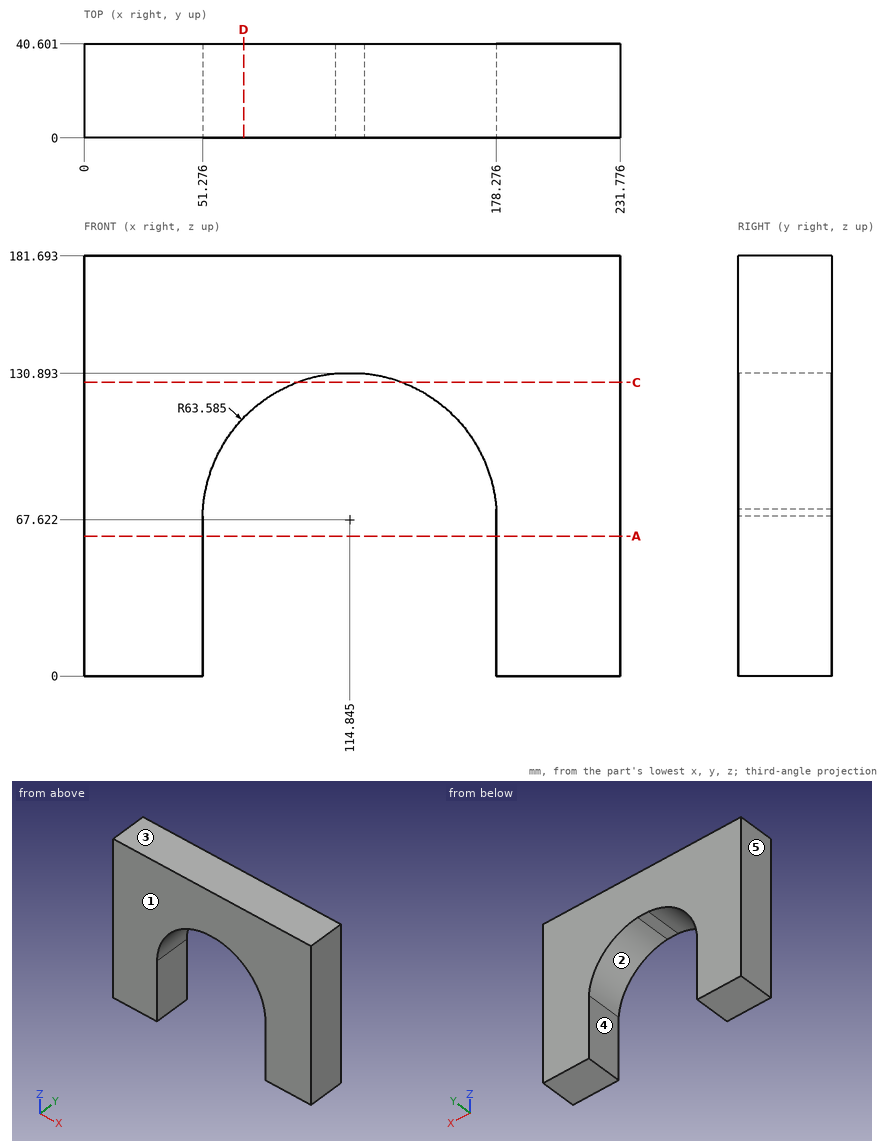
Drawing for the job (mm, zero at the part's lowest x, y, z). A direction names the side the tool comes from. Round coordinates to 2 decimals unless told otherwise and drop trailing zeros. Loops run counter-clockwise (first coordinate to the right, second up) from the corner with the lowest first, then second, coordinate; pieces in that order, holes last.
1. Mould opens along X. For the marked faces 3, 4 and 5 say: +X half, -X half, draft (parallel to the pull), parting line (faces both ways), or undercut.
Check values:
face 3: draft
face 4: undercut
face 5: -X half
2. Drop flat-ended pins along their axis: P1, Ø4, axis at x = 113.5, y = 15, coming from the -Z side; P2, Ø6, axis at x = 66, y = 30, coming from the -Z side (1 decimal). Give the stop position or say it passes through.
Check values:
P1: stops at z = 130.89
P2: stops at z = 104.4
3. Wall check: probe 1 along X at (y, z) = (13.5, 38); probe 2 along X at (y, z) = (19, 113) (1 decimal); probe 3 along Z at (x, y) = (66, 35) (1 decimal). Give the ranges that are in metal, low to high.
Check values:
probe 1: x = 0 to 51.28, 178.28 to 231.78
probe 2: x = 0 to 70.3, 159.4 to 231.8
probe 3: z = 108.3 to 181.7
4. Band-saw the part on C-C, the plane z = 127. List the corners of the cut face in (x, y), and give its area (3 significant figures).
Check values:
outline: (0, 0) - (92.1, 0) - (92.1, 40.6) - (0, 40.6) - close; (137.59, 0) - (231.78, 0) - (231.78, 40.6) - (137.59, 40.6) - close
area: 7,560 mm2
5. Tool access for the marked faces 1 and 2: list every direction of +Z, -Z, +X, -X, +Y, -Y with a clear straight run to the whole face (end or side of a thin tool).
Check values:
face 1: +Z, -Z, +X, -X, -Y
face 2: -Z, +Y, -Y
6. Band-saw the part on A-A, the plane z = 60.5. List the corners of the cut face in (x, y).
Check values:
outline: (0, 0) - (51.28, 0) - (51.28, 40.6) - (0, 40.6) - close; (178.28, 0) - (231.78, 0) - (231.78, 40.6) - (178.28, 40.6) - close
7. Band-saw the part on D-D, the plane x = 69. List the corners of the cut face in (y, z), and give its area (3 significant figures).
Check values:
outline: (0, 111.68) - (40.6, 111.68) - (40.6, 181.69) - (0, 181.69) - close
area: 2,840 mm2
